```python
from build123d import *

# Parameters (mm, degrees)
SKETCH_1_R      = 2.69
SKETCH_1_R_2    = 2
EXTRUDE_1_DEPTH = 0.77
SKETCH_2_R      = 3.95
SKETCH_2_R_2    = 2
EXTRUDE_2_DEPTH = 2
FILLET_1_R      = 0.2


with BuildPart() as part:
    # 草图1 → 凸台-拉伸1 (new body)
    with BuildSketch(Plane(origin=(0, 0, 0), x_dir=(1, 0, 0), z_dir=(0, 1, 0))):
        with Locations(Location((0, 0, 0), (0, 0, 270))):
            Circle(SKETCH_1_R)
        with Locations(Location((0, 0, 0), (0, 0, 270))):
            Circle(SKETCH_1_R_2, mode=Mode.SUBTRACT)
    extrude(amount=EXTRUDE_1_DEPTH)

    # 草图2 → 凸台-拉伸2 (add)
    with BuildSketch(Plane(origin=(0, 0.77, 0), x_dir=(1, 0, 0), z_dir=(0, 1, 0))):
        with Locations(Location((0, 0, 0), (0, 0, 270))):
            Circle(SKETCH_2_R)
        with Locations(Location((0, 0, 0), (0, 0, 270))):
            Circle(SKETCH_2_R_2, mode=Mode.SUBTRACT)
    extrude(amount=EXTRUDE_2_DEPTH)

    # 圆角1
    fillet_1_edges = [part.edges().sort_by_distance(p)[0] for p in [
        (0, 0.77, -3.95),
        (0, 2.77, -2),
        (0, 0, -2),
        (0, 2.77, -3.95),
    ]]
    fillet(fillet_1_edges, radius=FILLET_1_R)


solid = part.part
```
Read the model definition and answer for the solid it produces. Units are mm, in the model's axes. A direction names the side the tool comes from. Coordinates: 2 decimals unless noted, no trailing zeros. Write each loop counter-clockwise with the first axis right and the second up, starting at its lowest first coordinate (ties: lowest second). Pieces come first, ordered by that corner, then holes. Notation, with made-up numbers: (26, 39) -> (61, 39) arc R23 cw to (61, 52) -> close; hole circle Ø6 at (55.25, 14). An arc over 180 degrees is marked (long way). Return JSON: item names as keys, results as strings.
1. A tool of negligible diameter and unlimited length cuts with its end or side. For faces 1 (the face through (3, 0.77, -1)), 2 (the face through (-2, 2.77, 2)), from which of +Z, -Z, +X, -X, +Y, -Y can it reach the whole face along a straight path? Write none if from no direction.
Found:
{"face 1": "-Y", "face 2": "+Z, -Z, +X, -X, +Y"}
2. Find the intervals of material crossed by line 1 along X through (y, z) = (1.2, 0); line 2 along X through (y, z) = (1.85, 0.5); line 3 along Y through (x, z) = (2, 2.5), in increasing order. Write a range as from..to.
Found:
{"line 1": "-3.95..-2, 2..3.95", "line 2": "-3.92..-1.94, 1.94..3.92", "line 3": "0.77..2.77"}
3. A cutting plane is placed at A-A (x = 0). Determine the outline of the cut face in (y, z).
Found:
{"outline": "(0, -2.69) -> (0.77, -2.69) -> (0.77, -3.75) arc R0.2 ccw to (0.97, -3.95) -> (2.57, -3.95) arc R0.2 ccw to (2.77, -3.75) -> (2.77, -2.2) arc R0.2 ccw to (2.57, -2) -> (0.2, -2) arc R0.2 ccw to (0, -2.2) -> close; (0, 2.2) arc R0.2 ccw to (0.2, 2) -> (2.57, 2) arc R0.2 ccw to (2.77, 2.2) -> (2.77, 3.75) arc R0.2 ccw to (2.57, 3.95) -> (0.97, 3.95) arc R0.2 ccw to (0.77, 3.75) -> (0.77, 2.69) -> (0, 2.69) -> close"}
4. Each of these flat-tipped pins is pushed along its axis until it touches: P1, Ø1.5, axis at x = -2, y = 1.5, coming from the +Z side; P2, Ø1, axis at x = 1.5, z = 3, coming from the -Y side; P3, Ø1.5, axis at y = 1, z = -1.5, coming from the -X side. Where does it stop, or does it pass through?
Found:
{"P1": "z = 3.75", "P2": "y = 0.77", "P3": "x = -3.88"}
5. A cutting plane is placed at B-B (z = 0). Determine the outline of the cut face in (x, y), and give its area (3 significant figures).
Found:
{"outline": "(-3.95, 0.97) arc R0.2 ccw to (-3.75, 0.77) -> (-2.69, 0.77) -> (-2.69, 0) -> (-2.2, 0) arc R0.2 ccw to (-2, 0.2) -> (-2, 2.57) arc R0.2 ccw to (-2.2, 2.77) -> (-3.75, 2.77) arc R0.2 ccw to (-3.95, 2.57) -> close; (2, 0.2) arc R0.2 ccw to (2.2, 0) -> (2.69, 0) -> (2.69, 0.77) -> (3.75, 0.77) arc R0.2 ccw to (3.95, 0.97) -> (3.95, 2.57) arc R0.2 ccw to (3.75, 2.77) -> (2.2, 2.77) arc R0.2 ccw to (2, 2.57) -> close", "area": "8.79 mm2"}
6. A cutting plane is placed at C-C (y = 1.2). Determine the outline of the cut face in (x, z).
Found:
{"outline": "circle Ø7.9 at (0, 0); hole circle Ø4 at (0, 0)"}
